For this review, take the finished solid that the model builds, in its own axes (mm). Face numbers are marked on the shaded views. Coordinates: 2 decimals unless noted, no trailing zeros. Write each loop counter-clockwise with the first axis right and the second up, starting at its lowest first coordinate (ties: lowest second). Pieces come first, ordered by that corner, then holes. Notation, with made-up numbers: (49.25, 3) -> (58.25, 3) arc R11 ccw to (58.25, 24) -> close; hole circle Ø3 at (18, 23). An arc over 180 degrees is marked (long way). One line per item, written item: value. Start each with the question number.
1) Mouldability with a two-part tool opening along X and no side actions: class the marked faces 1, 2 and 3 as released by +X, released by -X, zero draft, split by the parting line, or undercut.
2) For probe 1 along Y at (x, z) = (-2, -8.5); probe 2 along X at (y, z) = (1.5, -1.75), list the stretches that pass through material, from the lowest coordinate up. Write a range as from..to.
3) Add section A-A (z = -21.5). State the section outline as (x, y) points.
4) For pin 1 Ø3 at (x, z) = (-2.5, -6) entering from -Y; pin 2 Ø3 at (y, z) = (-1, -9.5) entering from -X, all flat-tipped, find the tip position at first contact; note any pin that passes through.
Autodesk Inventor part; units mm, degrees
ref_plane "MSC_PF1" through (0, 0, 0) normal (1, 0, 0) x (0, 1, 0)
ref_plane "MSC_PT1" through (0, 0, 0) normal (0, 0, -1) x (-1, 0, 0)
ref_plane "YZ Plane" through (0, 0, 0) normal (1, 0, 0) x (0, 1, 0)
sketch "Szkic1" plane through (0, 0, 0) normal (0, 1, 0) x (-1, 0, 0)
  point P0 (0, 0)
sketch "Szkic2" plane through (0, 0, 0) normal (0, 1, 0) x (-1, 0, 0)
  line L0 (-2.5, -25) -> (0, -25)
  line L1 (-2.5, -2.8) -> (-2.5, -25)
  line L2 (-5, -0.3) -> (-2.5, -2.8)
  line L3 (-5, 0) -> (-5, -0.3)
  line L4 (0, 0) -> (-5, 0)
  line L5 (0, -25) -> (0, 0)
  line L6 (0, -25) -> (0, 0)
  line L7 (0, -30) -> (0, 5)
  line L8 (1, 0) -> (-6, 0)
  dimension "d3" = 5
  dimension "d5" = 2.5
  dimension "d7" = 25
  dimension "ParC" = 0.3
  dimension "d22" = 0
  dimension "d23" = 0
  dimension "d43" = 45
revolve "Obrót1" add sketch "Szkic2" angle 360 about axis through (0, 0, -25) along (0, 0, -1)
sketch "Szkic3" plane through (0, 0, 0) normal (0, 0, 1) x (1, 0, 0)
  line L0 (-1.5, 0.866) -> (-1.5, -0.866)
  line L1 (0, 1.7321) -> (-1.5, 0.866)
  line L2 (1.5, 0.866) -> (0, 1.7321)
  line L3 (1.5, -0.866) -> (1.5, 0.866)
  line L4 (0, -1.7321) -> (1.5, -0.866)
  line L5 (-1.5, -0.866) -> (0, -1.7321)
  circle A0 centre (0, 0) radius 1.5 construction
  circle A1 centre (0, 0) radius 2.5 construction
  dimension "d11" = 3
  dimension "d13" = 120
  dimension "d15" = 120
extrude "Wyciągnięcie proste1" cut sketch "Szkic3" against normal blind 2.3
fillet "Zaokrąglenie1" radius 0.2 1 edges at (-2.5, 0, -2.8)
chamfer "Faza1" distance 0.4 angle 45 1 edges at (-2.5, 0, -25) measured on face at (-0.599, -2.4272, -17.6276)
thread "Gwint1"
ref_plane "MSC_PF1" through (0, 0, 0) normal (1, 0, 0) x (0, 1, 0)
ref_plane "MSC_PT1" through (0, 0, 0) normal (0, 0, -1) x (-1, 0, 0)
equation "\"d3\" = 0.5 * dk"
equation "\"d5\" = 0.5 * NND"
equation "\"d7\" = NLG"
equation "\"d43\" = 0.5 * ang"
equation "\"d11\" = ParS"
equation "\"d16\" = ParT"
equation "\"d18\" = r"
equation "\"d19\" = 0.5 * PTC"
equation "\"d39\" = 0.5 * PTC"
equation "\"NND\" = 5"
equation "\"PTC\" = 0.8"
equation "\"ParK\" = 2.8"
equation "\"ParS\" = 3"
equation "\"ParT\" = 2.3"
equation "\"r\" = 0.2"
equation "\"NLG\" = 25"
equation "\"ang\" = 90deg"
equation "\"THREADDIA\" = NND"
properties part number "DIN 7991 - M5x25" material "Stal, miękka"
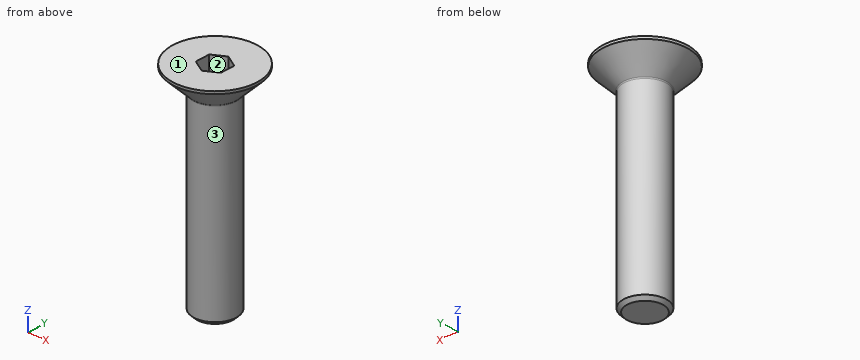
Numbers:
1. face 1: zero draft
1. face 2: undercut
1. face 3: split by the parting line
2. probe 1: -1.5..1.5
2. probe 2: -3.22..-0.4, 0.4..3.22
3. outline: circle Ø5 at (0, 0)
4. pin 1: y = -2.29
4. pin 2: x = -2.5
